Read the model definition and answer for the solid it produces. Units are mm, in the model's axes. A direction names the side the tool comes from. Coordinates: 2 decimals unless noted, no trailing zeros. Loops run counter-clockwise (first coordinate to the right, second up) from the corner with the lowest first, then second, coordinate; pieces in that order, holes last. Notation, with made-up numbers: (50, 88) - (87, 88) arc R21 ccw to (87, 106) - close; hole circle Ø5 at (-36.75, 37.5). An arc over 180 degrees is marked (long way). Use CSV: the item, a comma, the result in double quotes.
```python
from build123d import *

# Parameters (mm, degrees)
SKETCH1_R                       = 10.16
GEAR_SLOT_DEPTH                 = 12.7
CIRPATTERN1_COUNT               = 2
CIRPATTERN1_ANGLE               = 10
CIRPATTERN1_THE_OTHER_WAY_COUNT = 2
CIRPATTERN1_THE_OTHER_WAY_ANGLE = 10
GAS_MANIFOLD_DEPTH              = 7.62
FILLET1_R                       = 3.175
TAP_DRILL_FOR_10_32_TAP1_D      = 4.0386
TAP_DRILL_FOR_10_32_TAP1_DEPTH  = 17.836682152
TAP_DRILL_FOR_10_32_TAP1_TIP    = 1.213317848


with BuildPart() as part:
    # Sketch9 → Revolve1 (revolve)
    with BuildSketch(Plane.XY, mode=Mode.PRIVATE) as revolve1_sk:
        Polygon((-10.16, 10.16), (-10.16, 27.305), (-88.9, 27.305), (-88.9, -10.795), (-80.645, -10.795), (-80.645, 10.795), (-69.85, 10.795), (-69.85, 5.08), (-58.42, 5.08), (-58.42, 6.35), (-45.72, 6.35), (-45.72, 7.62), (-33.02, 7.62), (-33.02, 10.16), align=None)
    revolve(revolve1_sk.sketch.rotate(Axis((0, 18.1216542, 0), (0, -1, 0)), 270), axis=Axis((0, 18.1216542, 0), (0, -1, 0)))

    # Sketch1 → Gear Slot (cut)
    with BuildSketch(Plane(origin=(0, 27.305, 0), x_dir=(1, 0, 0), z_dir=(0, 1, 0))):
        with BuildLine():
            Line((62.5, -40.675), (79.049063087, -40.675))
            ThreePointArc((79.049063087, -40.675), (88.9, 0), (79.049063087, 40.675))
            Line((79.049063087, 40.675), (62.5, 40.675))
            ThreePointArc((62.5, 40.675), (58.41179797, 40.469028023), (54.365, 39.853198115))
            Line((54.365, 39.853198115), (-5.635, 27.605749401))
            ThreePointArc((-5.635, 27.605749401), (-28.175, 0), (-5.635, -27.605749401))
            Line((-5.635, -27.605749401), (54.365, -39.853198115))
            ThreePointArc((54.365, -39.853198115), (58.41179797, -40.469028023), (62.5, -40.675))
        make_face()
        with Locations(Location((0, 0, 0), (0, 0, 270))):
            Circle(SKETCH1_R, mode=Mode.SUBTRACT)
    extrude(amount=-GEAR_SLOT_DEPTH, mode=Mode.SUBTRACT)

    # Sketch5 one side → Orifice (revolve, cut)
    with BuildSketch(Plane(origin=(-76.2, 0, 0), x_dir=(0, 0, -1), z_dir=(1, 0, 0)), mode=Mode.PRIVATE) as orifice_sk:
        Polygon((-10.063777286, 15.998459659), (-7.555019185, 3.092018098), (-2.67011422, 5.474545442), (-10.464353209, 21.455103585), (-12.290702712, 20.564333415), align=None)
    orifice = revolve(orifice_sk.sketch.rotate(Axis((-76.2, 5.474545442, 2.67011422), (0, 0.8987940462991696, 0.43837114678907213)), 180), axis=Axis((-76.2, 5.474545442, 2.67011422), (0, 0.8987940462991696, 0.43837114678907213)), mode=Mode.SUBTRACT)

    # CirPattern1: Orifice ×2 about axis
    cirpattern1_axis = Axis((0, 17.78, 0), (0, -1, 0))
    for i in range(1, CIRPATTERN1_COUNT):
        add(orifice.rotate(cirpattern1_axis, i * CIRPATTERN1_ANGLE / (CIRPATTERN1_COUNT - 1)), mode=Mode.SUBTRACT)

    # CirPattern1 the other way: Orifice ×2 about axis
    cirpattern1_the_other_way_axis = Axis((0, 17.78, 0), (0, 1, 0))
    for i in range(1, CIRPATTERN1_THE_OTHER_WAY_COUNT):
        add(orifice.rotate(cirpattern1_the_other_way_axis, i * CIRPATTERN1_THE_OTHER_WAY_ANGLE / (CIRPATTERN1_THE_OTHER_WAY_COUNT - 1)), mode=Mode.SUBTRACT)

    # Sketch10 → Gas Manifold (cut)
    with BuildSketch(Plane(origin=(0, 27.305, 0), x_dir=(1, 0, 0), z_dir=(0, 1, 0))):
        with BuildLine():
            ThreePointArc((-65.637529562, -23.890107011), (-69.85, 0), (-65.637529562, 23.890107011))
            ThreePointArc((-65.637529562, 23.890107011), (-69.432749794, 32.028983063), (-77.571625846, 28.233762832))
            ThreePointArc((-77.571625846, 28.233762832), (-82.55, 0), (-77.571625846, -28.233762832))
            ThreePointArc((-77.571625846, -28.233762832), (-69.432749794, -32.028983063), (-65.637529562, -23.890107011))
        make_face()
    extrude(amount=-GAS_MANIFOLD_DEPTH, mode=Mode.SUBTRACT)

    # Fillet1
    fillet1_edges = [part.edges().sort_by_distance(p)[0] for p in [
        (79.049063087, 20.955, -40.675),
        (79.049063087, 20.955, 40.675),
    ]]
    fillet(fillet1_edges, radius=FILLET1_R)

    # Tap Drill for #10-32 Tap1
    with Locations(Plane(origin=(44.901280605, 27.305, -44.901280605), x_dir=(0, 0, 1), z_dir=(0, 1, 0))):
        with Locations((0, 0), (-12.649263872, -71.737540226), (102.451825082, -71.737540226), (89.80256121, 0)):
            Hole(TAP_DRILL_FOR_10_32_TAP1_D / 2, depth=TAP_DRILL_FOR_10_32_TAP1_DEPTH)
            with Locations((0, 0, -(TAP_DRILL_FOR_10_32_TAP1_DEPTH + TAP_DRILL_FOR_10_32_TAP1_TIP / 2))):  # 118° drill point
                Cone(0, TAP_DRILL_FOR_10_32_TAP1_D / 2, TAP_DRILL_FOR_10_32_TAP1_TIP, mode=Mode.SUBTRACT)


solid = part.part
```
Q1. A tool of negligible diameter and unlimited length cuts with its end or side. For faces 4 (the face through (-13.8, 7.62, 30.3)), 5 (the face through (-79.37, 6.86, 17.52)), 6 (the face through (68, 21, 40.675)), from which of +Z, -Z, +X, -X, +Y, -Y can it reach the whole face along a straight path? Write none if from no direction.
Reported:
face 4,"-Y"
face 5,"none"
face 6,"+X, +Y"
Q2. The part is cut by section C-C on z = 72.5. Determine the outline of the cut face in (x, y) (3 decimals), and give its area (3 significant figures).
Reported:
outline,"(-51.449, -10.795) - (-35.318, -10.795) - (-35.318, 10.795) - (35.318, 10.795) - (35.318, -10.795) - (51.449, -10.795) - (51.449, 27.305) - (-51.449, 27.305) - close"
area,"2,400 mm²"
Q3. The part is cut by section B-B on y = 24. Determine the outline of the cut face in (x, z) (3 decimals), and give its area (3 significant figures).
Reported:
outline,"(-5.635, -27.606) arc R28.175 cw to (-5.635, 27.606) - (54.365, 39.853) arc R40.675 cw to (62.5, 40.675) - (73.661, 40.675) arc R3.175 ccw to (76.389, 45.474) arc R88.9 ccw (long way) to (76.389, -45.474) arc R3.175 ccw to (73.661, -40.675) - (62.5, -40.675) arc R40.675 cw to (54.365, -39.853) - close; hole (-77.572, -28.234) arc R6.35 ccw to (-65.638, -23.89) arc R69.85 cw to (-65.638, 23.89) arc R6.35 ccw to (-77.572, 28.234) arc R82.55 ccw to start; hole circle Ø4.039 at (-26.836, -57.551); hole circle Ø4.039 at (-26.836, 57.551); hole circle Ø4.039 at (44.901, -44.901); hole circle Ø4.039 at (44.901, 44.901)"
area,"16,400 mm²"
Q4. Find the intervals of material crossed by probe 1 along X at (y, z) = (5.9, 0) (3 decimals); probe 2 along X at (y, z) = (5, 0) (3 decimals); probe 3 along Y at (x, z) = (-23, 49.5) (3 decimals), in increasing order. Write a range as [from, to].
Reported:
probe 1,"x = [-88.9, -80.645], [-69.85, -58.42], [58.42, 69.85], [80.645, 88.9]"
probe 2,"x = [-88.9, -80.645], [80.645, 88.9]"
probe 3,"y = [6.35, 27.305]"
Q5. The part is cut by section D-D on x = -18.5. Determine the outline of the cut face in (y, z) (3 decimals), and give its area (3 significant figures).
Reported:
outline,"(-10.795, -86.954) - (27.305, -86.954) - (27.305, -21.25) - (14.605, -21.25) - (14.605, 21.25) - (27.305, 21.25) - (27.305, 86.954) - (-10.795, 86.954) - (-10.795, 78.494) - (10.795, 78.494) - (10.795, 67.356) - (5.08, 67.356) - (5.08, 55.413) - (6.35, 55.413) - (6.35, 41.81) - (7.62, 41.81) - (7.62, 27.351) - (10.16, 27.351) - (10.16, -27.351) - (7.62, -27.351) - (7.62, -41.81) - (6.35, -41.81) - (6.35, -55.413) - (5.08, -55.413) - (5.08, -67.356) - (10.795, -67.356) - (10.795, -78.494) - (-10.795, -78.494) - close"
area,"3,080 mm²"
Q6. Given P1, Ø6.5, axis at x = -26.84, z = 57.55, coming from the +Y side (3 decimals); P2, Ø6, axis at x = 42.5, y = -2, coming from the +Z side; P3, Ø10, axis at x = 57.5, y = 2.5, coming from the -Z side; P4, Ø2.5, axis at x = 44.9, z = 44.9, coming from the -Y side, each flat-ended and moving along its own axis, determine where each tip first touches the part or whether it passes through.
Reported:
P1,"stops at y = 27.305"
P2,"stops at z = 79.64"
P3,"stops at z = -71.74"
P4,"stops at y = 5.08"
Q7. For a pull along Y with two mould halves and no side action, classify faces 1 (the face through (-81.205, 6.863, 3.471)), 2 (the face through (7, 10.16, -8)), 3 (the face through (-82.55, 23.55, -0.4)) as +Y half, -Y half, draft (parallel to the pull), parting line (faces both ways), or undercut.
Reported:
face 1,"undercut"
face 2,"-Y half"
face 3,"draft"
